Build history of the part. All positions in model axes, mm. Face numbers are marked on the shaded views. A direction names the side the tool comes from. Give positions to 0.01 mm unless a question says otherwise; leave off trailing zeros. Loops run counter-clockwise (first coordinate to the right, second up) from the corner with the lowest first, then second, coordinate; pieces in that order, holes last. Notation, with made-up numbers: M 78.5,-8.5 L 95.5,-8.5 A16 cw 95.5,6.5 Z; hole C -30.5,53.25 d2. An arc over 180 degrees is marked long. Put each result on its own line as item: value.
```python
from build123d import *

# Parameters (mm, degrees)
SKETCH_1_W          = 55
SKETCH_1_H          = 36.8
EXTRUDE_1_DEPTH     = 4
SKETCH_2_W          = 40
SKETCH_2_H          = 36.8
EXTRUDE_2_DEPTH     = 20
SKETCH_3_W          = 40
SKETCH_3_H          = 2
CUT_EXTRUDE_1_DEPTH = 200
SKETCH_4_R          = 2.1
CUT_EXTRUDE_2_DEPTH = 200
SKETCH_5_R          = 7.591855359
EXTRUDE_3_DEPTH     = 15


with BuildPart() as part:
    # 草图1 → 凸台-拉伸1 (new body)
    with BuildSketch(Plane(origin=(0, 0, 0), x_dir=(1, 0, 0), z_dir=(0, 1, 0))):
        Rectangle(SKETCH_1_W, SKETCH_1_H)
    extrude(amount=EXTRUDE_1_DEPTH)

    # 草图2 → 凸台-拉伸2 (add)
    with BuildSketch(Plane(origin=(0, 4, 0), x_dir=(1, 0, 0), z_dir=(0, 1, 0))):
        Rectangle(SKETCH_2_W, SKETCH_2_H)
    extrude(amount=EXTRUDE_2_DEPTH)

    # 草图3 → 切除-拉伸1 (cut)
    with BuildSketch(Plane.XY.offset(18.4)):
        Rectangle(SKETCH_3_W, SKETCH_3_H)
    extrude(amount=-CUT_EXTRUDE_1_DEPTH, mode=Mode.SUBTRACT)

    # 草图4 → 切除-拉伸2 (cut)
    with BuildSketch(Plane(origin=(0, 4, 0), x_dir=(1, 0, 0), z_dir=(0, 1, 0))):
        with Locations(Location((-23.95, 0, 0), (0, 0, 270))):
            Circle(SKETCH_4_R)
        with Locations(Location((23.95, 14.35, 0), (0, 0, 270))):
            Circle(SKETCH_4_R)
        with Locations(Location((23.95, -14.35, 0), (0, 0, 270))):
            Circle(SKETCH_4_R)
    extrude(amount=-CUT_EXTRUDE_2_DEPTH, mode=Mode.SUBTRACT)

    # 草图5 → 凸台-拉伸3 (add)
    with BuildSketch(Plane(origin=(20, 0, 0), x_dir=(0, 0, -1), z_dir=(1, 0, 0))):
        with Locations(Location((0, 13.214422917, 0), (0, 0, 180))):
            Circle(SKETCH_5_R)
    extrude(amount=EXTRUDE_3_DEPTH)


solid = part.part
```
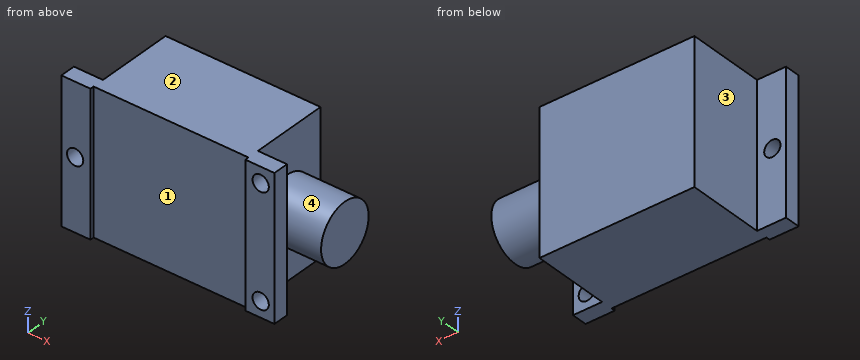
Q1. Slice it at C-C (x = 25). List the corners of the cut face in (y, z).
Here are the results:
outline: M 0,-18.4 L 4,-18.4 L 4,-16.17 L 0,-16.17 Z; M 0,-12.53 L 4,-12.53 L 4,12.53 L 0,12.53 Z; M 0,16.17 L 4,16.17 L 4,18.4 L 0,18.4 Z; C 13.21,0 d15.18
Q2. Tool access for the marked faces 1, 2, 3 and 4: list every direction of +Z, -Z, +X, -X, +Y, -Y with a clear straight run to the whole face (end or side of a thin tool).
Here are the results:
face 1: +Z, -Z, -Y
face 2: +Z, +X, -X, +Y, -Y
face 3: +Z, -Z, -X, +Y
face 4: +X
Q3. Slice it at D-D (y = 15.75). List the corners of the cut face in (x, z), and give its area (3 significant figures).
Here are the results:
outline: M -20,-18.4 L 20,-18.4 L 20,-7.16 L 35,-7.16 L 35,7.16 L 20,7.16 L 20,18.4 L -20,18.4 Z
area: 1,690 mm²
Q4. Probe line 1 (X direction, y = 2.4, z = 14.35); line 2 (X direction, y = 2.05, z = 0); line 3 (Y direction, x = 22, z = -13). List the from-to ranges inside material, lowest first. Write a range as from..to.
Here are the results:
line 1: -27.5..21.85, 26.05..27.5
line 2: -27.5..-26.05, -21.85..27.5
line 3: 0..4
Q5. Slice it at A-A (x = -23.95). List the corners of the cut face in (y, z), and give its area (3 significant figures).
Here are the results:
outline: M 0,-18.4 L 4,-18.4 L 4,-2.1 L 0,-2.1 Z; M 0,2.1 L 4,2.1 L 4,18.4 L 0,18.4 Z
area: 130 mm²
Q6. Drop flat-ended pins along their axis: pin 1 Ø5 at (y, z) = (6, -9) entering from +X; pin 2 Ø6 at (y, z) = (15, 8.5) entering from -X; pin 3 Ø2 at (x, z) = (16.5, 2) entering from -Y. Give the stop position or say it passes through.
Here are the results:
pin 1: x = 27.5
pin 2: x = -20
pin 3: y = 1
Q7. Slice it at B-B (z = -14.35). List the corners of the cut face in (x, y), and give its area (3 significant figures).
Here are the results:
outline: M -27.5,0 L -20,0 L -20,1 L 20,1 L 20,0 L 21.85,0 L 21.85,4 L 20,4 L 20,24 L -20,24 L -20,4 L -27.5,4 Z; M 26.05,0 L 27.5,0 L 27.5,4 L 26.05,4 Z
area: 963 mm²
